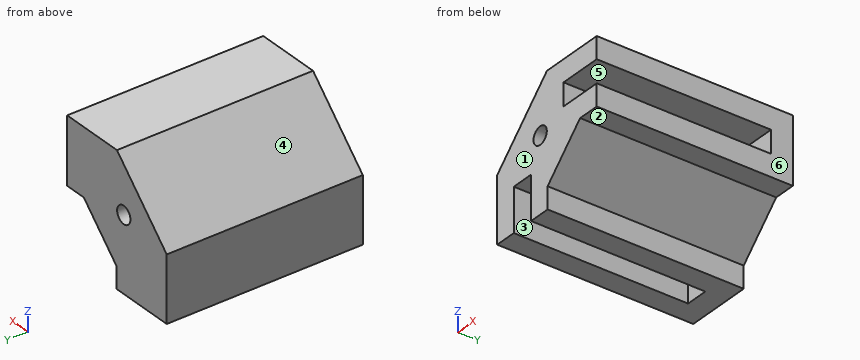
```python
from build123d import *

# Parameters (mm, degrees)
BOSS_EXTRUDE1_DEPTH         = 50.8
TAP_DRILL_FOR_1_4_20_TAP1_D = 5.08
SKETCH4_R                   = 2.54
BOSS_EXTRUDE2_DEPTH         = 6.35


with BuildPart() as part:
    # Sketch1 → Boss-Extrude1 (new body)
    with BuildSketch(Plane(origin=(0, 0, 0), x_dir=(1, 0, 0), z_dir=(0, 1, 0))):
        Polygon((22.098, 9.652), (9.652, 22.098), (9.652, 28.448), (3.302, 28.448), (3.302, 15.748), (-3.302, 15.748), (-3.302, 28.448), (-9.652, 28.448), (-9.652, 9.398), (9.398, -9.652), (28.448, -9.652), (28.448, -3.302), (15.748, -3.302), (15.748, 3.302), (28.448, 3.302), (28.448, 9.652), align=None)
    extrude(amount=BOSS_EXTRUDE1_DEPTH)

    # Tap Drill for 1/4-20 Tap1 (through all)
    with Locations(Plane(origin=(0, 50.8, 0), x_dir=(1, 0, 0), z_dir=(0, 1, 0))):
        with Locations((6.795346667, 6.795346667)):
            Hole(TAP_DRILL_FOR_1_4_20_TAP1_D / 2)

    # Sketch4 → Boss-Extrude2 (add)
    with BuildSketch(Plane(origin=(0, 50.8, 0), x_dir=(1, 0, 0), z_dir=(0, 1, 0))):
        Polygon((-3.302, 28.448), (3.302, 28.448), (9.652, 28.448), (9.652, 22.098), (22.098, 9.652), (28.448, 9.652), (28.448, 3.302), (28.448, -3.302), (28.448, -9.652), (9.398, -9.652), (-9.652, 9.398), (-9.652, 28.448), align=None)
        with Locations(Location((6.795346667, 6.795346667, 0), (0, 0, 270))):
            Circle(SKETCH4_R, mode=Mode.SUBTRACT)
    extrude(amount=BOSS_EXTRUDE2_DEPTH)


solid = part.part
```
Input: part model. Units: mm. Frame: model coordinates. Face numbers are marked on the shaded views. A direction names the side the tool comes from. Round coordinates to 2 decimals unless told otherwise and drop trailing zeros. Loops run counter-clockwise (first coordinate to the right, second up) from the corner with the lowest first, then second, coordinate; pieces in that order, holes last. Notation, with made-up numbers: M -26.75,87.5 L -8.75,87.5 A19 cw -8.75,95.5 Z; hole C 59,78 d3. An arc over 180 degrees is marked long. Answer in a Markdown table with one row per item. Add a question column.
1. Section A-A (x = 19). Output: boundary loops of the cut face in (y, z), and give its area (3 significant figures).
2. Section B-B (z = -16.5). Output: boundary loops of the cut face in (x, y).
3. Section C-C (y = 14). Output: boundary loops of the cut face in (x, z), and give its area (3 significant figures).
4. Ray query, probe 1 along Z at (x, y) = (23, 4); probe 2 along X at (y, z) = (18.5, -6). Return the intervals inside material, ascending.
5. Section D-D (x = 0.5). Output: boundary loops of the cut face in (y, z), and give its area (3 significant figures).
6. Contact query for flat-ended pins moving along their axis: pin 1 (2 mm diameter, centred on y = 19.5, z = 0, fed in from +X); pin 2 (2 mm diameter, centred on x = 8, y = 44, fed in from +Z); pin 3 (3 mm diameter, centred on x = 1, y = 45, fed in from -Z). Output: stop coordinate, or through.
7. Mould query, pull axis Z, two halves, no side actions, for the marked faces 4, 5 and 6. Classes: released by +Z, released by -Z, zero draft, split by the parting line, or undercut.
8. Set-up query: the marked faces 1, 2 and 3. Return all of +Z, -Z, +X, -X, +Y, -Y with unobstructed straight access to the full face (end or side cutting, diameter ignored); none if empty.
Values follow:
| question | item | result |
|---|---|---|
| 1 | outline | M 0,-12.75 L 57.15,-12.75 L 57.15,9.65 L 0,9.65 L 0,3.3 L 50.8,3.3 L 50.8,-3.3 L 0,-3.3 Z |
| 1 | area | 945 mm^2 |
| 2 | outline | M -9.65,0 L -3.3,0 L -3.3,50.8 L 3.3,50.8 L 3.3,0 L 15.25,0 L 15.25,57.15 L -9.65,57.15 Z |
| 3 | outline | M -9.65,-28.45 L -3.3,-28.45 L -3.3,-15.75 L 3.3,-15.75 L 3.3,-28.45 L 9.65,-28.45 L 9.65,-22.1 L 22.1,-9.65 L 28.45,-9.65 L 28.45,-3.3 L 15.75,-3.3 L 15.75,3.3 L 28.45,3.3 L 28.45,9.65 L 9.4,9.65 L -9.65,-9.4 Z; hole C 6.8,-6.8 d5.08 |
| 3 | area | 806 mm^2 |
| 4 | probe 1 | -9.65 to -3.3, 3.3 to 9.65 |
| 4 | probe 2 | -6.25 to 4.38, 9.21 to 28.45 |
| 5 | outline | M 0,-15.75 L 50.8,-15.75 L 50.8,-28.45 L 57.15,-28.45 L 57.15,0.75 L 0,0.75 Z |
| 5 | area | 1,020 mm^2 |
| 6 | pin 1 | x = 15.75 |
| 6 | pin 2 | z = 9.25 |
| 6 | pin 3 | z = -15.75 |
| 7 | face 4 | released by +Z |
| 7 | face 5 | undercut |
| 7 | face 6 | zero draft |
| 8 | face 1 | +Z, -Z, +X, -X, -Y |
| 8 | face 2 | -Z, +X, +Y, -Y |
| 8 | face 3 | -Z, -Y |
